```python
from build123d import *

# Parameters (mm, degrees)
SKETCH3_W           = 17.8
SKETCH3_H           = 16
BOSS_EXTRUDE1_DEPTH = 1.2
BOSS_EXTRUDE2_DEPTH = 0.4


with BuildPart() as part:
    # Sketch2 → Revolve1 (revolve)
    with BuildSketch(Plane(origin=(0, 0, 0), x_dir=(1, 0, 0), z_dir=(0, 1, 0))):
        with BuildLine():
            Line((0, -8), (-8, -8))
            Line((-8, -8), (-8, 6.6))
            Line((-8, 6.6), (-6.5, 6.8))
            Line((-6.5, 6.8), (-6.5, 26.35))
            ThreePointArc((-6.5, 26.35), (-6.133883476, 27.233883476), (-5.25, 27.6))
            Line((-5.25, 27.6), (-1, 27.6))
            Line((-1, 27.6), (-1, 31.6))
            Line((-1, 31.6), (0, 31.6))
            Line((0, 31.6), (0, -8))
        make_face()
    revolve(axis=Axis((0, 0, 8), (0, 0, -1)))

    # Sketch3 → Boss-Extrude1 (add)
    with BuildSketch(Plane.XY):
        with Locations((-8.9, 0)):
            Rectangle(SKETCH3_W, SKETCH3_H)
    extrude(amount=-BOSS_EXTRUDE1_DEPTH)

    # Sketch5 → Boss-Extrude2 (add, symmetric)
    with BuildSketch(Plane(origin=(0, 0, 0), x_dir=(1, 0, 0), z_dir=(0, 1, 0))):
        Polygon((-2, 30.2), (2, 30.2), (3.5, 31.859853002), (3.5, 40.540146998), (2, 42.2), (-2, 42.2), (-3.5, 40.540146998), (-3.5, 31.859853002), align=None)
    extrude(amount=BOSS_EXTRUDE2_DEPTH, both=True)


solid = part.part
```
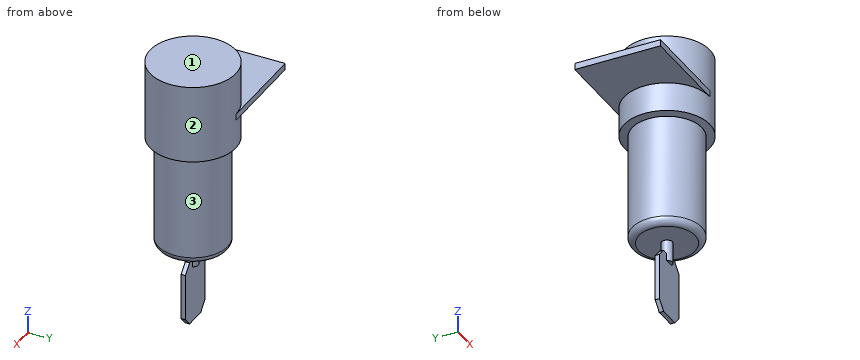
The model under review builds one solid part; all positions refer to its coordinate system, in mm. Face numbers are marked on the shaded views. A direction names the side the tool comes from. Round coordinates to 2 decimals unless told otherwise and drop trailing zeros. Loops run counter-clockwise (first coordinate to the right, second up) from the corner with the lowest first, then second, coordinate; pieces in that order, holes last. Notation, with made-up numbers: (-10, 51.5) -> (29, 51.5) arc R30 ccw to (29, 86.5) -> close; hole circle Ø5 at (29.25, -10.75). An arc over 180 degrees is marked (long way). Answer as a JSON object with one key per item and string values. Group by question number.
1) For pin 1 Ø2 at (x, y) = (-13, 4.5) entering from -Z; pin 2 Ø0.6 at (y, z) = (0, -38) entering from -X; pin 3 Ø0.5 at (x, y) = (-0.5, -1) entering from -Z, all flat-tipped, find the tip position at first contact; note any pin that passes through.
2) We need section A-A on z = 1. Write out the cut boundary in (x, y), then the cut area to 3 significant figures.
3) For line 1 (Z direction, x = -16.25, y = -3); line 2 (Z direction, x = 4.5, y = -2.75); line 3 (Y direction, x = -2.25, z = -36.5), list the stretches that pass through material, from the lowest coordinate up. Write a range as [from, to].
4) For the marked faces 1, 2 and 3, list the 3-axis set-ups (+Z, -Z, +X, -X, +Y, -Y) from which the entire face can be reached by the end or side of a thin tool; tool diameter is ignored.
Result set:
{
 "1": {"pin 1": "z = -1.2", "pin 2": "x = -3.5", "pin 3": "z = -31.6"},
 "2": {"outline": "circle Ø16 at (0, 0)", "area": "201 mm²"},
 "3": {"line 1": "[-1.2, 0]", "line 2": "[-27.6, 8]", "line 3": "[-0.4, 0.4]"},
 "4": {"face 1": "+Z, +X, -X, +Y, -Y", "face 2": "none", "face 3": "-Z"}
}
